Input: dimensioned drawing with shaded views. Units: mm. Origin: part minimum x, y, z. A direction names the side the tool comes from. Coordinates: 2 decimals unless noted, no trailing zeros. Loops run counter-clockwise (first coordinate to the right, second up) from the corner with the lowest first, then second, coordinate; pieces in that order, holes last. Notation, with made-up numbers: (72.25, 89.5) -> (106.25, 89.5) arc R23 ccw to (106.25, 126.5) -> close; hole circle Ø9 at (31.5, -32). An arc over 180 degrees is marked (long way). Answer as CSV lines item,"result".
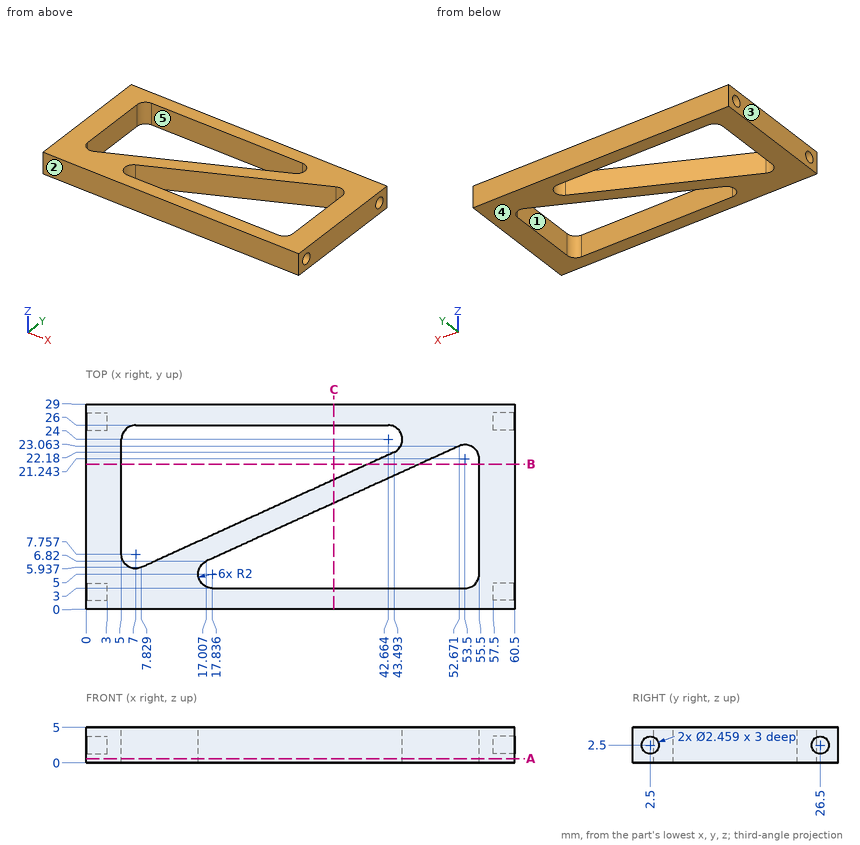
(1) Material intervals for L1, parallel to Y at x = 58.5, z = 2.5; L2, parallel to Y at x = 17.5, z = 0.55 (1 decimal); L3, parallel to Y at x = 53.5, z = 4.6, sorted ascending. Write a range as [from, to].
Computed values:
L1,"[0, 1.27], [3.73, 25.27], [27.73, 29]"
L2,"[0, 3], [7, 10.3], [26, 29]"
L3,"[0, 3], [23.24, 29]"
(2) Cut plane C-C (x = 35). Return the cut outline in (y, z) (1 decimal).
Computed values:
outline,"(0, 0) -> (3, 0) -> (3, 5) -> (0, 5) -> close; (15, 0) -> (18.3, 0) -> (18.3, 5) -> (15, 5) -> close; (26, 0) -> (29, 0) -> (29, 5) -> (26, 5) -> close"
(3) Pin query (flat end, axial travel): pin 1 Ø1.5 at (y, z) = (2.5, 2.5) entering from +X; pin 2 Ø1.2 at (y, z) = (2.5, 2) entering from -X. Return the tip coordinate at first contact, or that it passes through.
Computed values:
pin 1,"x = 57.5"
pin 2,"x = 3"
(4) Draft query along X for the marked faces 1, 2 and 3. Return one class per face: released by +X, released by -X, zero draft, split by the parting line, or undercut.
Computed values:
face 1,"undercut"
face 2,"zero draft"
face 3,"released by -X"
(5) Cut plane A-A (z = 0.6). Return the cut outline in (x, y) (1 decimal).
Computed values:
outline,"(0, 0) -> (60.5, 0) -> (60.5, 29) -> (0, 29) -> close; hole (5, 7.8) arc R2 ccw to (7.8, 5.9) -> (43.5, 22.2) arc R2 ccw to (42.7, 26) -> (7, 26) arc R2 ccw to (5, 24) -> close; hole (17, 6.8) arc R2 ccw to (17.8, 3) -> (53.5, 3) arc R2 ccw to (55.5, 5) -> (55.5, 21.2) arc R2 ccw to (52.7, 23.1) -> close"
(6) Access query for the marked faces 4 and 5. Directions: +Z, -Z, +X, -X, +Y, -Y. A direction counts if a zero-diameter tool reaches every point of the face in a straight line with its end or side. Return the directions, or none.
Computed values:
face 4,"-Z, +X, -X, +Y, -Y"
face 5,"+Z, -Z"
(7) Cut plane B-B (y = 20.5). Return the cut outline in (x, z) (1 decimal).
Computed values:
outline,"(0, 0) -> (5, 0) -> (5, 5) -> (0, 5) -> close; (39.8, 0) -> (47, 0) -> (47, 5) -> (39.8, 5) -> close; (55.5, 0) -> (60.5, 0) -> (60.5, 5) -> (55.5, 5) -> close"
